Here's how the part is built. I have some questions about the finished solid (model axes, mm). A direction names the side the tool comes from. Round coordinates to 2 decimals unless told otherwise and drop trailing zeros. Write each loop counter-clockwise with the first axis right and the second up, starting at its lowest first coordinate (ties: lowest second). Pieces come first, ordered by that corner, then holes. Notation, with made-up numbers: (85, -15) - (131, -15) arc R19 ccw to (131, 12) - close; hole circle Ø11 at (10, -22.5). An arc over 180 degrees is marked (long way). One line per item, written item: value. Start each with the question number.
Item 1: Thinking about a two-plate mould opening in Y: for faces 6 (the face through (0.3, 7.5, -9.35)), 7 (the face through (0, 2.6, 8)), 8 (the face through (0.33, 6.51, -8.86)), which applies, released by +Y, released by -Y, zero draft, split by the parting line, or undercut?
Item 2: Imagine slicing it at C-C, the plane z = -2.75. Please give me the cut outline in (x, y).
Item 3: Imagine slicing it at A-A, the plane x = -17.5. Please give me the cut outline in (y, z), then the cut area to 3 significant figures.
Item 4: For P1, Ø4, axis at y = 0, z = 9.5, coming from the -X side; P2, Ø8, axis at x = 17.5, y = 0, coming from the -Z side; P3, Ø4, axis at y = -1, z = 9, coming from the +X side, each with a flat end and sliding along its axis, tell me the tip position at first contact or that it passes through.
Item 5: If I drill on line 1 (Y direction, x = -17.5, z = -3); line 2 (Y direction, x = 16, z = -0.25); line 3 (X direction, y = 1.25, z = -2), over which ranges is the centre line in solid material (lowest first)?
Item 6: Imagine slicing it at D-D, the plane x = 6. Please give me the cut outline in (y, z).
Item 7: For faces 1 (the face through (23.5, 0, -1)), 2 (the face through (0, -2.6, 8)), 3 (the face through (4.5, 0, 9)), 4 (the face through (0, -6, -8)), 5 (the face through (0.06, 2.09, 10.66)), which set-ups out of +Z, -Z, +X, -X, +Y, -Y let a thin tool reach every point of the face, with its end or its side?
Item 8: Imagine slicing it at B-B, the plane y = 0. Please give me the cut outline in (x, z), then the cut area to 4 significant figures.
Autodesk Inventor part; units mm, degrees
ref_plane "YZ Plane" through (0, 0, 0) normal (1, 0, 0) x (0, 1, 0)
ref_plane "XZ Plane" through (0, 0, 0) normal (0, 1, 0) x (-1, 0, 0)
ref_plane "XY Plane" through (0, 0, 0) normal (0, 0, 1) x (1, 0, 0)
ref_plane "작업 평면1" through (23.5, -8, -2) normal (1, 0, 0) x (0, 0, -1)
sketch "스케치1" plane through (23.5, -8, -2) normal (1, 0, 0) x (0, 0, -1)
  line L0 (0, 16) -> (-8.15, 16)
  line L1 (-8.15, 16) -> (-8.15, 10.6)
  line L2 (-8.15, 10.6) -> (-12.15, 10.6)
  line L3 (-13.15, 9.6) -> (-12.15, 10.6)
  line L4 (-13.15, 9.6) -> (-13.15, 6.4)
  line L5 (-12.15, 5.4) -> (-13.15, 6.4)
  line L6 (-12.15, 5.4) -> (-8.15, 5.4)
  line L7 (-8.15, 5.4) -> (-8.15, 0)
  line L8 (-8.15, 0) -> (0, 0)
  line L9 (0, 16) -> (7.35, 16)
  line L10 (7.35, 16) -> (7.35, 15)
  line L11 (7.35, 15) -> (6.35, 14)
  line L12 (5.35, 14) -> (5.35, 2)
  line L13 (5.35, 14) -> (6.35, 14)
  line L14 (0, 0) -> (7.35, 0)
  line L15 (7.35, 0) -> (7.35, 1)
  line L16 (7.35, 1) -> (6.35, 2)
  line L17 (5.35, 2) -> (6.35, 2)
  line L18 (0, 16) -> (-8.15, 16)
  line L19 (-8.15, 10.6) -> (-12.15, 10.6)
  line L20 (-8.15, 10.6) -> (-12.15, 10.6)
  line L21 (-12.15, 10.6) -> (-13.15, 9.6)
  line L22 (-13.15, 6.4) -> (-12.15, 5.4)
  point P0 (-2, 8)
  dimension "d1" = 7.35
sketch "스케치2" plane through (-23.5, 8, 6.15) normal (0, 0, 1) x (1, 0, 0)
  arc A0 (7.9209, -9.6) -> (7.9209, -6.4) centre (6, -8) ccw
  line L0 (39.0791, -9.6) -> (7.9209, -9.6)
  circle A1 centre (6, -8) radius 2.5
  circle A2 centre (41, -8) radius 2.5
  circle A3 centre (41, -8) radius 2.5
  point P0 (23.5, -8)
  point P1 (7.9209, -6.4)
extrude "돌출1" add sketch "스케치1" against normal up to surface (47 mm away)
extrude "돌출2" cut sketch "스케치2" along normal mid plane 50
sketch "스케치3" plane through (-15.5791, 1.6, 11.15) normal (0, 0, 1) x (1, 0, 0)
  line L0 (15.5791, -14.4593) -> (15.5791, 15.5737)
  line L1 (-7.9209, 4.4) -> (-7.9209, -7.6)
  line L2 (-7.9209, 4.4) -> (11.0791, 4.4)
  line L3 (11.0791, 4.4) -> (11.0791, -7.6)
  line L4 (11.0791, -7.6) -> (-7.9209, -7.6)
  line L5 (-7.9209, -7.6) -> (-7.9209, 4.4)
  line L6 (39.0791, 4.4) -> (39.0791, -7.6)
  line L7 (39.0791, 4.4) -> (20.0791, 4.4)
  line L8 (20.0791, 4.4) -> (20.0791, -7.6)
  line L9 (20.0791, -7.6) -> (39.0791, -7.6)
  line L10 (39.0791, -7.6) -> (39.0791, 4.4)
  point P0 (15.5791, -1.6)
  dimension "d9" = 19
extrude "돌출3" cut sketch "스케치3" against normal up to surface (5 mm away)
sketch "스케치4" plane through (-23.5, 8, 6.15) normal (0, 0, 1) x (1, 0, 0)
  circle A0 centre (6, -8) radius 2.5
  circle A1 centre (6, -8) radius 3
  circle A2 centre (41, -8) radius 2.5
  circle A3 centre (41, -8) radius 3
  point P0 (23.5, -8)
  dimension "d10" = 6
  dimension "d11" = 6
extrude "돌출4" cut sketch "스케치4" against normal up to surface (13.5 mm away) contours A0 | A1 | A2 | A3
properties part number "Bearing Spacer_1mmUP"
Values follow:
1. face 6: zero draft
1. face 7: released by +Y
1. face 8: undercut
2. outline: (-23.5, -8) - (23.5, -8) - (23.5, 8) - (-23.5, 8) - close; hole circle Ø6 at (-17.5, 0); hole circle Ø6 at (17.5, 0)
3. outline: (-8, -9.35) - (-7, -9.35) - (-6, -8.35) - (-6, -7.35) - (-3, -7.35) - (-3, 6.15) - (-8, 6.15) - close; (3, -7.35) - (6, -7.35) - (6, -8.35) - (7, -9.35) - (8, -9.35) - (8, 6.15) - (3, 6.15) - close
3. area: 142 mm^2
4. P1: stops at x = -4.5
4. P2: stops at z = -7.35
4. P3: stops at x = 4.5
5. line 1: y = -8 to -3, 3 to 8
5. line 2: y = -8 to -2.6, 2.6 to 8
5. line 3: x = -23.5 to -20.23, -14.77 to 14.77, 20.23 to 23.5
6. outline: (-8, -9.35) - (-7, -9.35) - (-6, -8.35) - (-6, -7.35) - (6, -7.35) - (6, -8.35) - (7, -9.35) - (8, -9.35) - (8, 6.15) - (-8, 6.15) - close
7. face 1: +Z, -Z, +X, +Y, -Y
7. face 2: +Z, +X, -X, -Y
7. face 3: +Z, +X, +Y, -Y
7. face 4: -Z, +X, -X
7. face 5: +Z, +X, -X, +Y
8. outline: (-23.5, -7.35) - (-20.5, -7.35) - (-20.5, 6.15) - (-23.5, 6.15) - close; (-14.5, -7.35) - (14.5, -7.35) - (14.5, 6.15) - (4.5, 6.15) - (4.5, 11.15) - (-4.5, 11.15) - (-4.5, 6.15) - (-14.5, 6.15) - close; (20.5, -7.35) - (23.5, -7.35) - (23.5, 6.15) - (20.5, 6.15) - close
8. area: 517.5 mm^2
